from build123d import *


with BuildPart() as part:
    # Sweep2: sweep along a path in Sketch4
    with BuildLine(Plane(origin=(0, 0, 0), x_dir=(1, 0, 0), z_dir=(0, 1, 0))) as sweep2_path:
        Line((0, 0), (0, 240))
        Line((0, 240), (-240, 240))
    # Sketch3 → Sweep2 (sweep)
    with BuildSketch(Plane.XY):
        Polygon((0, -4.442807786), (0, -24.442807786), (20, -24.442807786), (20, -9.442807786), (14.811670364, -14.631137422), (9.811670364, -9.631137422), (15, -4.442807786), align=None)
    sweep(path=sweep2_path.line, transition=Transition.RIGHT)


solid = part.part
Geometry check sheet. Reference: the model listing, model coordinates, mm. A direction names the side the tool comes from. Round coordinates to 2 decimals unless told otherwise and drop trailing zeros. Write each loop counter-clockwise with the first axis right and the second up, starting at its lowest first coordinate (ties: lowest second). Pieces come first, ordered by that corner, then holes.
Item 1: Access from +Z, -Z, +X, -X, +Y, -Y to the whole of each face (thin tool, end or side, straight path). Record for faces 1 (the face through (-53, -24.443, -246)), 2 (the face through (0, -14, -122)).
Determined:
face 1: +Z, -Z, +X, -X, -Y
face 2: +Z, -X, +Y, -Y
Item 2: Section check B-B (z = -58). Record the boundary of the cut face in (x, y), plus the area to 3 significant figures.
Determined:
outline: (0, -24.44) - (20, -24.44) - (20, -9.44) - (14.81, -14.63) - (9.81, -9.63) - (15, -4.44) - (0, -4.44) - close
area: 336 mm2
Item 3: Section check C-C (y = -18.5). Record the boundary of the cut face in (x, z).
Determined:
outline: (-240, -260) - (20, -260) - (20, 0) - (0, 0) - (0, -240) - (-240, -240) - close
Item 4: Material ranges on line 1 along X through (y, z) = (-21, -148); line 2 along Z through (x, y) = (-128, -18); line 3 along X through (y, z) = (-10.5, -106), recorded low to high.
Determined:
line 1: x = 0 to 20
line 2: z = -260 to -240
line 3: x = 0 to 10.68, 18.94 to 20
Item 5: Section check A-A (x = -45). Record the boundary of the cut face in (y, z), plus the area to 3 significant figures.
Determined:
outline: (-24.44, -260) - (-9.44, -260) - (-14.63, -254.81) - (-9.63, -249.81) - (-4.44, -255) - (-4.44, -240) - (-24.44, -240) - close
area: 336 mm2
Item 6: Go/stop test with flat-tipped pins: pin 1 Ø8 at (x, y) = (-43.5, -15) entering from +Z; pin 2 Ø1 at (y, z) = (-12.5, -210.5) entering from -X. Record where each tip stops, or that it passes through.
Determined:
pin 1: stops at z = -240
pin 2: stops at x = 0
